Autodesk Inventor part; units mm, degrees
ref_plane "Start Plane" through (0, 0, 17.9725) normal (0, 0, 1) x (1, 0, 0)
ref_plane "End Plane" through (0, 0, 991.1616) normal (0, 0, 1) x (1, 0, 0)
ref_plane "Work Plane4" through (-23.8819, -0.0809, 32.329) normal (-0.2481, 0.0809, -0.9653) x (-0.7765, 0.5792, 0.2481)
ref_plane "Start Plane" through (0, 0, 17.9725) normal (0, 0, 1) x (1, 0, 0)
ref_plane "End Plane" through (0, 0, 991.1616) normal (0, 0, 1) x (1, 0, 0)
sketch "Sketch" plane through (0, 0, 0) normal (0, 0, 1) x (1, 0, 0)
  circle A0 centre (0, 0) radius 20.447
  circle A1 centre (0, 0) radius 24.13
  dimension "d0" = 48.26
  dimension "d1" = 3.683
extrude "Body" add sketch "Sketch" along normal up to surface (973.1891 mm away) from surface at 17.9725
sketch "Sketch3" plane through (0, 0, 0) normal (0, 0, 1) x (1, 0, 0)
  line L0 (0, 0) -> (10, 0)
ref_plane "Work Plane3" through (0, 0, 0) normal (0, -1, 0) x (1, 0, 0)
ref_plane "Work Plane4" through (-23.8819, -0.0809, 32.329) normal (-0.2481, 0.0809, -0.9653) x (-0.7765, 0.5792, 0.2481)
split "Split1" plane through (-23.8819, -0.0809, 32.329) removes the side toward (-0.2481, 0.0809, -0.9653)
ref_plane "Work Plane5" through (6.5041, 0, 986.4388) normal (-0.2588, 0, 0.9659) x (0.9659, 0, 0.2588)
split "Split2" plane through (6.5041, 0, 986.4388) removes the side toward (-0.2588, 0, 0.9659)
sketch "Sketch4" plane through (0, 0, 0) normal (0, -1, 0) x (1, 0, 0)
  line L0 (-2, 17.9725) -> (12, 17.9725)
  line L1 (-2, 991.1616) -> (12, 991.1616)
  dimension "d7" = 973.189
equation "\"d0\" = G_H"
equation "\"d1\" = G_T"
equation "\"d2\" = G_L"
equation "\"G_H\" = 48.26"
equation "\"G_T\" = 3.683"
equation "\"G_L\" = d7"
equation "\"G_OFFSET_START\" = -17.97254"
equation "\"G_OFFSET_END\" = -19.55088"
equation "\"d4\" = -G_OFFSET_START"
equation "\"d5\" = G_OFFSET_END + B_L"
equation "\"B_L\" = 1010.71247"
properties part number "ANSI - 1 1/2 x 0.145 - 38.315" material "Steel, Mild"
For this review, take the finished solid that the model builds, in its own axes (mm). Give positions to 0.01 mm unless a question says otherwise; leave off trailing zeros. Write each loop counter-clockwise with the first axis right and the second up, starting at its lowest first coordinate (ties: lowest second). Pieces come first, ordered by that corner, then holes. Notation, with made-up numbers: M -22,1.5 L -3,1.5 A33 ccw -3,35.5 Z; hole C 76,72.5 d2. An arc over 180 degrees is marked long. Answer as a JSON object with one key per item and string values. Group by question number.
Item 1: Consider section C-C on z = 321. Write out the cut boundary in (x, y), plus the area to 3 significant figures.
Item 2: Draft analysis for pull direction Y (two halves, no side actions). For faces 1 (the cylindrical face through (23.016, -7.248, 498.575)), 2 (the cylindrical face through (19.503, -6.142, 498.601)), 3 (the flat face through (12.4, 16.47, 24.39)), state which applies: +Y half, -Y half, draft (parallel to the pull), parting line (faces both ways), or undercut.
Item 3: For pin 1 Ø3 at (x, z) = (9.5, 628.5) entering from +Y; pin 2 Ø3 at (x, y) = (18, -4) entering from -Z; pin 3 Ø12 at (x, z) = (-9, 269.5) entering from -Y; pin 4 Ø2 at (y, z) = (1.5, 660.5) entering from +X, all flat-tipped, find the tip position at first contact; note any pin that passes through.
Item 4: Consider section B-B on x = 11. Write out the cut boundary in (y, z) (3 decimals), plus the area to 3 significant figures.
Item 5: For probe 1 along X at (y, z) = (0, 434); probe 2 along Y at (x, z) = (18.5, 594.5), list the stretches that pass through material, from the lowest coordinate up. Write a range as [from, to].
Item 6: Consider section A-A on y = -11.5. Write out the cut boundary in (x, z), plus the area to 3 significant figures.
Check result:
{
 "1": {"outline": "C 0,0 d48.26; hole C 0,0 d40.89", "area": "516 mm^2"},
 "2": {"face 1": "parting line", "face 2": "undercut", "face 3": "+Y half"},
 "3": {"pin 1": "stops at y = 22.77", "pin 2": "passes through", "pin 3": "stops at y = -23.94", "pin 4": "stops at x = 24.12"},
 "4": {"outline": "M -21.477,21.571 L -17.236,21.926 L -17.236,987.643 L -21.477,987.643 Z; M 17.236,24.815 L 21.477,25.17 L 21.477,987.643 L 17.236,987.643 Z", "area": "8,180 mm^2"},
 "5": {"probe 1": "x = [-24.13, -20.45], [20.45, 24.13]", "probe 2": "y = [-15.49, -8.71], [8.71, 15.49]"},
 "6": {"outline": "M -21.21,30.69 L -16.91,29.58 L -16.91,980.17 L -21.21,979.01 Z; M 16.91,20.89 L 21.21,19.78 L 21.21,990.38 L 16.91,989.23 Z", "area": "8,260 mm^2"}
}
